Can you work these out from the model? Positions are in its coordinate system, mm. Give positions to 0.01 mm unless a question says otherwise; leave off trailing zeros. Return JSON: item names as keys, results as strings. Group by question number.
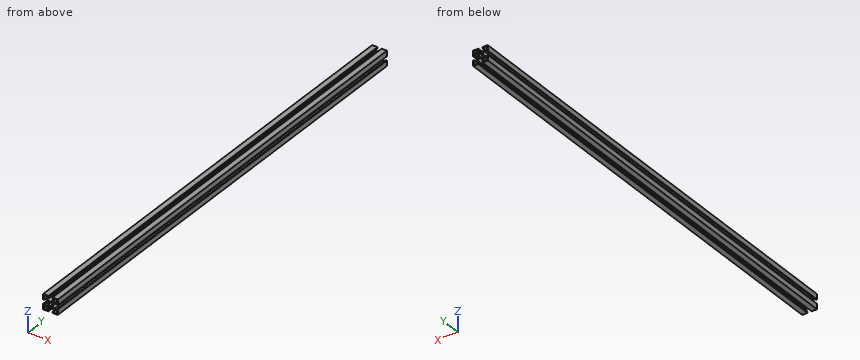
from build123d import *

# Parameters (mm, degrees)
F0_R     = 2
F0_R_2   = 2.15
F1_DEPTH = 312


# Not quite as in the source:
# - ends of sketch curves that miss each other by under 0.0002 mm in the source are joined


with BuildPart() as f1:
    # F0 (on Front) → F1 (new body, symmetric)
    with BuildSketch(Plane.XZ):
        with BuildLine():
            Line((4.49119, 14.509531), (4.49119, 11.252281))
            ThreePointArc((4.49119, 11.252281), (4.4613472004, 11.1218391084), (4.377756086, 11.0173488916))
            ThreePointArc((4.377756086, 11.0173488916), (2.6232116259, 10.0239112371), (0.6484679813, 9.6168093955))
            Line((0.6484679813, 9.6168093955), (0.34119, 9.309531))
            Line((0.34119, 9.309531), (0.033913, 9.616809))
            ThreePointArc((0.033913, 9.616809), (-1.9408311583, 10.0239110615), (-3.695375823, 11.0173492229))
            ThreePointArc((-3.695375823, 11.0173492229), (-3.7789672004, 11.1218391084), (-3.80881, 11.252281))
            Line((-3.80881, 11.252281), (-3.80881, 14.509531))
            ThreePointArc((-3.80881, 14.509531), (-3.7209420344, 14.7216630344), (-3.50881, 14.809531))
            Line((-3.50881, 14.809531), (-2.60881, 14.809531))
            ThreePointArc((-2.60881, 14.809531), (-2.3966779656, 14.8973989656), (-2.30881, 15.109531))
            Line((-2.30881, 15.109531), (-2.30881, 16.009531))
            ThreePointArc((-2.30881, 16.009531), (-2.3966779656, 16.2216630344), (-2.60881, 16.309531))
            Line((-2.60881, 16.309531), (-9.35881, 16.309531))
            ThreePointArc((-9.35881, 16.309531), (-9.5709420344, 16.2216630344), (-9.65881, 16.009531))
            Line((-9.65881, 16.009531), (-9.65881, 9.259531))
            ThreePointArc((-9.65881, 9.259531), (-9.5709420344, 9.0473989656), (-9.35881, 8.959531))
            Line((-9.35881, 8.959531), (-8.45881, 8.959531))
            ThreePointArc((-8.45881, 8.959531), (-8.2466779656, 9.0473989656), (-8.15881, 9.259531))
            Line((-8.15881, 9.259531), (-8.15881, 10.159531))
            ThreePointArc((-8.15881, 10.159531), (-8.0709420344, 10.3716630344), (-7.85881, 10.459531))
            Line((-7.85881, 10.459531), (-4.601559, 10.459531))
            ThreePointArc((-4.601559, 10.459531), (-4.471117461, 10.4296883706), (-4.3666273786, 10.3460976993))
            ThreePointArc((-4.3666273786, 10.3460976993), (-3.3731893747, 8.5915529924), (-2.9660873955, 6.6168089813))
            Line((-2.9660873955, 6.6168089813), (-2.65881, 6.309531))
            Line((-2.65881, 6.309531), (-2.966087, 6.002254))
            ThreePointArc((-2.966087, 6.002254), (-3.3731890615, 4.0275098417), (-4.3666272229, 2.272965177))
            ThreePointArc((-4.3666272229, 2.272965177), (-4.4711171084, 2.1893737996), (-4.601559, 2.159531))
            Line((-4.601559, 2.159531), (-7.85881, 2.159531))
            ThreePointArc((-7.85881, 2.159531), (-8.0709420344, 2.2473989656), (-8.15881, 2.459531))
            Line((-8.15881, 2.459531), (-8.15881, 3.359531))
            ThreePointArc((-8.15881, 3.359531), (-8.2466779656, 3.5716630344), (-8.45881, 3.659531))
            Line((-8.45881, 3.659531), (-9.35881, 3.659531))
            ThreePointArc((-9.35881, 3.659531), (-9.5709420344, 3.5716630344), (-9.65881, 3.359531))
            Line((-9.65881, 3.359531), (-9.65881, -3.390469))
            ThreePointArc((-9.65881, -3.390469), (-9.5709420344, -3.6026010344), (-9.35881, -3.690469))
            Line((-9.35881, -3.690469), (-2.60881, -3.690469))
            ThreePointArc((-2.60881, -3.690469), (-2.3966779656, -3.6026010344), (-2.30881, -3.390469))
            Line((-2.30881, -3.390469), (-2.30881, -2.490469))
            ThreePointArc((-2.30881, -2.490469), (-2.3966779656, -2.2783369656), (-2.60881, -2.190469))
            Line((-2.60881, -2.190469), (-3.50881, -2.190469))
            ThreePointArc((-3.50881, -2.190469), (-3.7209420344, -2.1026010344), (-3.80881, -1.890469))
            Line((-3.80881, -1.890469), (-3.80881, 1.366782))
            ThreePointArc((-3.80881, 1.366782), (-3.7789672004, 1.4972238916), (-3.695376086, 1.6017141084))
            ThreePointArc((-3.695376086, 1.6017141084), (-1.9408311583, 2.5951519385), (0.0339130165, 3.0022536517))
            Line((0.0339130165, 3.0022536517), (0.34119, 3.309531))
            Line((0.34119, 3.309531), (0.648468, 3.002254))
            ThreePointArc((0.648468, 3.002254), (2.6232116259, 2.5951517629), (4.377755823, 1.6017137771))
            ThreePointArc((4.377755823, 1.6017137771), (4.4613472004, 1.4972238916), (4.49119, 1.366782))
            Line((4.49119, 1.366782), (4.49119, -1.890469))
            ThreePointArc((4.49119, -1.890469), (4.4033220344, -2.1026010344), (4.19119, -2.190469))
            Line((4.19119, -2.190469), (3.29119, -2.190469))
            ThreePointArc((3.29119, -2.190469), (3.0790579656, -2.2783369656), (2.99119, -2.490469))
            Line((2.99119, -2.490469), (2.99119, -3.390469))
            ThreePointArc((2.99119, -3.390469), (3.0790579656, -3.6026010344), (3.29119, -3.690469))
            Line((3.29119, -3.690469), (10.04119, -3.690469))
            ThreePointArc((10.04119, -3.690469), (10.2533220344, -3.6026010344), (10.34119, -3.390469))
            Line((10.34119, -3.390469), (10.34119, 3.359531))
            ThreePointArc((10.34119, 3.359531), (10.2533220344, 3.5716630344), (10.04119, 3.659531))
            Line((10.04119, 3.659531), (9.14119, 3.659531))
            ThreePointArc((9.14119, 3.659531), (8.9290579656, 3.5716630344), (8.84119, 3.359531))
            Line((8.84119, 3.359531), (8.84119, 2.459531))
            ThreePointArc((8.84119, 2.459531), (8.7533220344, 2.2473989656), (8.54119, 2.159531))
            Line((8.54119, 2.159531), (5.28394, 2.159531))
            ThreePointArc((5.28394, 2.159531), (5.1534981084, 2.1893737996), (5.0490078916, 2.272964914))
            ThreePointArc((5.0490078916, 2.272964914), (4.0555700615, 4.0275098417), (3.6484683483, 6.0022540165))
            Line((3.6484683483, 6.0022540165), (3.34119, 6.309531))
            Line((3.34119, 6.309531), (3.648468, 6.616809))
            ThreePointArc((3.648468, 6.616809), (4.0555703747, 8.5915529924), (5.0490087099, 10.3460974363))
            ThreePointArc((5.0490087099, 10.3460974363), (5.153498461, 10.4296883706), (5.28394, 10.459531))
            Line((5.28394, 10.459531), (8.54119, 10.459531))
            ThreePointArc((8.54119, 10.459531), (8.7533220344, 10.3716630344), (8.84119, 10.159531))
            Line((8.84119, 10.159531), (8.84119, 9.259531))
            ThreePointArc((8.84119, 9.259531), (8.9290579656, 9.0473989656), (9.14119, 8.959531))
            Line((9.14119, 8.959531), (10.04119, 8.959531))
            ThreePointArc((10.04119, 8.959531), (10.2533220344, 9.0473989656), (10.34119, 9.259531))
            Line((10.34119, 9.259531), (10.34119, 16.009531))
            ThreePointArc((10.34119, 16.009531), (10.2533220344, 16.2216630344), (10.04119, 16.309531))
            Line((10.04119, 16.309531), (3.29119, 16.309531))
            ThreePointArc((3.29119, 16.309531), (3.0790579656, 16.2216630344), (2.99119, 16.009531))
            Line((2.99119, 16.009531), (2.99119, 15.109531))
            ThreePointArc((2.99119, 15.109531), (3.0790579656, 14.8973989656), (3.29119, 14.809531))
            Line((3.29119, 14.809531), (4.19119, 14.809531))
            ThreePointArc((4.19119, 14.809531), (4.4033220344, 14.7216630344), (4.49119, 14.509531))
        make_face()
        with Locations((-6.65881, -0.690469)):
            Circle(F0_R, mode=Mode.SUBTRACT)
        with Locations((7.34119, -0.690469)):
            Circle(F0_R, mode=Mode.SUBTRACT)
        with Locations((-6.65881, 13.309531)):
            Circle(F0_R, mode=Mode.SUBTRACT)
        with Locations((0.34119, 6.309531)):
            Circle(F0_R_2, mode=Mode.SUBTRACT)
        with Locations((7.34119, 13.309531)):
            Circle(F0_R, mode=Mode.SUBTRACT)
    extrude(amount=F1_DEPTH, both=True)


solid = f1.part
1) I need wall thicknesses on line 1 along X through (y, z) = (138, 12.75); line 2 along Z through (x, y) = (-2.75, 51.5); line 3 along Z through (x, y) = (-7, -226). Which ranges of each line are inside material? Lowest first, please.
2) Will these pins go through, and if not, where does the flat tip stop? pin 1 Ø3 at (x, z) = (-6.66, -0.69) entering from +Y; pin 2 Ø2 at (y, z) = (-195, 7.5) entering from -X.
3) Imagine slicing it at A-A, the plane y = -204.5. Count the separate pieces of the cut face and the enclosed holes in it, and give its area (3 significant figures).
Resolved:
{
 "1": {"line 1": "-9.66 to -8.58, -4.74 to -3.81, 4.49 to 5.42, 9.26 to 10.34", "line 2": "-3.69 to -2.19, 2.23 to 6.22, 6.4 to 10.39, 14.81 to 16.31", "line 3": "-3.69 to -2.66, 1.28 to 2.16, 10.46 to 11.34, 15.28 to 16.31"},
 "2": {"pin 1": "through", "pin 2": "x = -3.34"},
 "3": {"separate pieces": "1", "enclosed holes": "5", "area": "146 mm^2"}
}
